Design review of the part shown in the three views and the two pictorial views. Dimensions are in mm from the part's minimum x, y and z. A direction names the side the tool comes from. Coordinates: 2 decimals unless noted, no trailing zeros. Loops run counter-clockwise (first coordinate to the right, second up) from the corner with the lowest first, then second, coordinate; pieces in that order, holes last. Notation, with made-up numbers: (3, 3.5) - (50, 3.5) arc R20 ccw to (50, 22.5) - close; hole circle Ø2 at (5.25, -22). An arc over 180 degrees is marked (long way). One line per item, written item: value. Start each with the question number.
1. Insertion check: pin 1 (1.6 mm diameter, centred on x = 10.5, z = 2.5, fed in from +Y); pin 2 (3 mm diameter, centred on y = 7.5, z = 1.5, fed in from -X); pin 3 (1.2 mm diameter, centred on x = 4.5, z = 1, fed in from -Y). Each pin has a flat end and moves straight along its axis. Give the tip position at first contact, or say it passes through.
2. For the marked faces 1 and 2, list the 3-axis set-ups (+Z, -Z, +X, -X, +Y, -Y) from which the entire face can be reached by the end or side of a thin tool; tool diameter is ignored.
3. Take a section at C-C, the plane x = 7.5. State the section outline as (y, z) points.
4. Take a section at A-A, the plane y = 7.5. State the section outline as (x, z) points, and give its area (3 significant figures).
5. Take a section at B-B, the plane z = 1.5. State the section outline as (x, y) points, and give its area (3 significant figures).
6. Take a section at D-D, the plane y = 1.5. State the section outline as (x, z) points.
7. To check wall thickness, follow line 1 (Y direction, x = 4.55, z = 1.5); line 2 (X direction, y = 13.7, z = 14); line 3 (X direction, y = 7.25, z = 17.25). State the ranges of each line that lie inside material, in increasing order. Write a range as from..to.
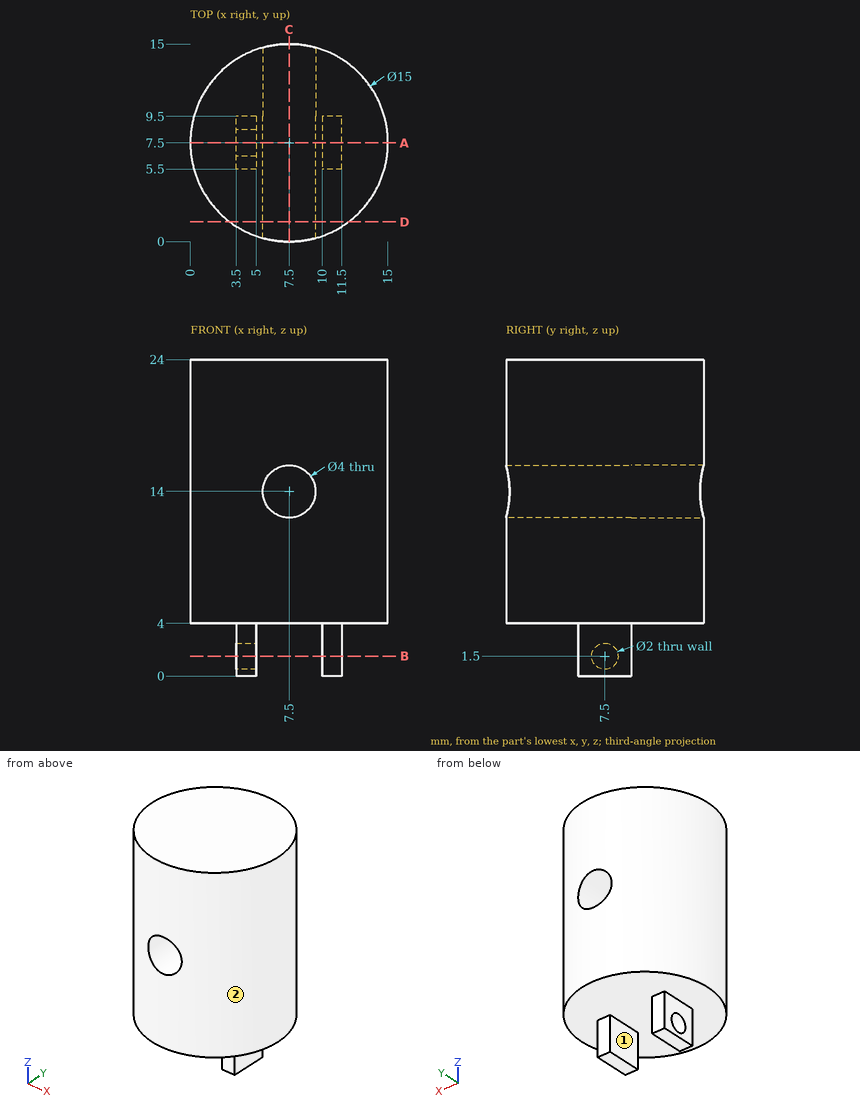
Solutions:
1. pin 1: y = 9.5
1. pin 2: x = 3.5
1. pin 3: y = 5.5
2. face 1: -Z, +Y, -Y
2. face 2: +Z, -Z
3. outline: (0, 4) - (15, 4) - (15, 12) - (0, 12) - close; (0, 16) - (15, 16) - (15, 24) - (0, 24) - close
4. outline: (0, 4) - (3.5, 4) - (3.5, 2.5) - (5, 2.5) - (5, 4) - (10, 4) - (10, 0) - (11.5, 0) - (11.5, 4) - (15, 4) - (15, 24) - (0, 24) - close; (3.5, 0) - (5, 0) - (5, 0.5) - (3.5, 0.5) - close; hole circle Ø4 at (7.5, 14)
4. area: 296 mm2
5. outline: (3.5, 5.5) - (5, 5.5) - (5, 6.5) - (3.5, 6.5) - close; (3.5, 8.5) - (5, 8.5) - (5, 9.5) - (3.5, 9.5) - close; (10, 5.5) - (11.5, 5.5) - (11.5, 9.5) - (10, 9.5) - close
5. area: 9.00 mm2
6. outline: (3, 4) - (12, 4) - (12, 24) - (3, 24) - close; hole circle Ø4 at (7.5, 14)
7. line 1: 5.5..6.5, 8.5..9.5
7. line 2: 3.28..5.5, 9.5..11.72
7. line 3: 0..15
